Part model, mm, in its own coordinate system. Face numbers are marked on the shaded views. A direction names the side the tool comes from. Coordinates: 2 decimals unless noted, no trailing zeros. Order: outer loops, then holes, each group sorted by start corner. A loop starts at its lowest first (then second) coordinate and runs counter-clockwise, first axis right, second up.
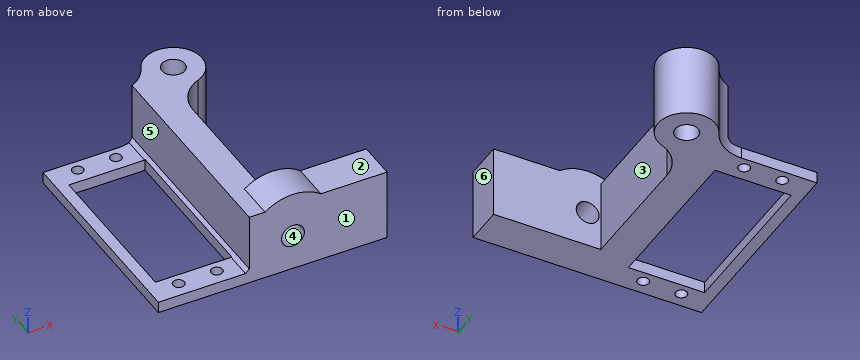
```python
from build123d import *

# Parameters (mm, degrees)
ESQUISSE1_W             = 60
ESQUISSE1_H             = 56
ESQUISSE1_W_2           = 20
ESQUISSE1_H_2           = 42
BOSS_EXTRU_1_DEPTH      = 3
ESQUISSE2_R             = 1.5
ENL_V_MAT_EXTRU_2_DEPTH = 83.127948958
BOSS_EXTRU_2_DEPTH      = 16
ESQUISSE4_W             = 28.138132954
ESQUISSE4_H             = 46
ENL_V_MAT_EXTRU_3_DEPTH = 84.618179841
ESQUISSE5_R             = 7.5
ESQUISSE5_R_2           = 3
BOSS_EXTRU_3_DEPTH      = 19
CONG_1_R                = 10
CONG_2_R                = 10
BOSS_EXTRU_4_DEPTH      = 10
ESQUISSE10_R            = 3
ENL_V_MAT_EXTRU_4_DEPTH = 10
CHANFREIN1_SIZE         = 1


with BuildPart() as part:
    # Esquisse1 → Boss.-Extru.1 (new body)
    with BuildSketch(Plane.XY):
        with Locations((30, 28)):
            Rectangle(ESQUISSE1_W, ESQUISSE1_H)
        with Locations((13, 28)):
            Rectangle(ESQUISSE1_W_2, ESQUISSE1_H_2, mode=Mode.SUBTRACT)
    extrude(amount=BOSS_EXTRU_1_DEPTH)

    # Esquisse2 → Enlèv. mat.-Extru.2 (cut, through all)
    with BuildSketch(Plane.XY.offset(3)):
        with Locations((7.5, 53)):
            Circle(ESQUISSE2_R)
        with Locations((17.5, 53)):
            Circle(ESQUISSE2_R)
        with Locations((7.5, 4)):
            Circle(ESQUISSE2_R)
        with Locations((17.5, 4)):
            Circle(ESQUISSE2_R)
    extrude(amount=-ENL_V_MAT_EXTRU_2_DEPTH, mode=Mode.SUBTRACT)

    # Esquisse3 → Boss.-Extru.2 (add)
    with BuildSketch(Plane.XY.offset(3)):
        Polygon((23.861867046, 56), (31.861867046, 56), (31.861867046, 10), (60, 10), (60, 0), (23.861867046, 0), align=None)
    extrude(amount=BOSS_EXTRU_2_DEPTH)

    # Esquisse4 → Enlèv. mat.-Extru.3 (cut, through all)
    with BuildSketch(Plane.XY.offset(3)):
        with Locations((45.930933523, 33)):
            Rectangle(ESQUISSE4_W, ESQUISSE4_H)
    extrude(amount=-ENL_V_MAT_EXTRU_3_DEPTH, mode=Mode.SUBTRACT)

    # Esquisse5 → Boss.-Extru.3 (add)
    with BuildSketch(Plane(origin=(0, 0, 0), x_dir=(-1, 0, 0), z_dir=(0, 0, -1))):
        with Locations((-35.561058301, 58.5)):
            Circle(ESQUISSE5_R)
        with Locations((-35.561058301, 58.5)):
            Circle(ESQUISSE5_R_2, mode=Mode.SUBTRACT)
    extrude(amount=-BOSS_EXTRU_3_DEPTH)

    # Congé1
    cong_1_edges = [part.edges().sort_by_distance(p)[0] for p in [
        (28.489990489, 56, 9.5),
    ]]
    fillet(cong_1_edges, radius=CONG_1_R)

    # Congé2
    cong_2_edges = [part.edges().sort_by_distance(p)[0] for p in [
        (31.861867046, 51.975738811, 9.5),
    ]]
    fillet(cong_2_edges, radius=CONG_2_R)

    # Esquisse9 → Boss.-Extru.4 (add)
    with BuildSketch(Plane.XZ):
        with BuildLine():
            Line((42.649653768, 19), (27.986775469, 19))
            ThreePointArc((27.986775469, 19), (35.318214618, 21.5), (42.649653768, 19))
        make_face()
    extrude(amount=-BOSS_EXTRU_4_DEPTH)

    # Esquisse10 → Enlèv. mat.-Extru.4 (cut)
    with BuildSketch(Plane.XZ):
        with Locations(Location((35.318214618, 9.5, 0), (0, 0, 270))):
            Circle(ESQUISSE10_R)
    extrude(amount=-ENL_V_MAT_EXTRU_4_DEPTH, mode=Mode.SUBTRACT)

    # Chanfrein1
    # the kernel refuses this chamfer: 1 mm, written as the material it adds along each edge
    with BuildSketch(Plane(origin=(23.861867046, 0, 3), x_dir=(0.027495876610585623, 0, 0.9996219169112968), z_dir=(0, 1, 0))) as chanfrein1_piece_1_section:
        Polygon((CHANFREIN1_SIZE * 0.999621916911, -CHANFREIN1_SIZE * 0.0274958766106), (-CHANFREIN1_SIZE * 0.0274958766106, -CHANFREIN1_SIZE * 0.999621916911), (0, 0), align=None)
    chanfrein1_piece_1 = extrude(amount=59.456320381, mode=Mode.PRIVATE)
    chanfrein1_piece_1 = split(chanfrein1_piece_1, bisect_by=Plane(origin=(23, 3.5, 3.33918952), z_dir=(1, 0, 0)), keep=Keep.TOP, mode=Mode.PRIVATE)
    chanfrein1_piece_1 = split(chanfrein1_piece_1, bisect_by=Plane(origin=(23.549970381, 7, 3.33918952), z_dir=(0, -1, 0)), keep=Keep.TOP, mode=Mode.PRIVATE)
    add(chanfrein1_piece_1)
    with BuildSketch(Plane(origin=(23.861867046, 0, 3), x_dir=(0.027495876610585623, 0, 0.9996219169112968), z_dir=(0, 1, 0))) as chanfrein1_piece_2_section:
        Polygon((CHANFREIN1_SIZE * 0.999621916911, -CHANFREIN1_SIZE * 0.0274958766106), (-CHANFREIN1_SIZE * 0.0274958766106, -CHANFREIN1_SIZE * 0.999621916911), (0, 0), align=None)
    chanfrein1_piece_2 = extrude(amount=59.456320381, mode=Mode.PRIVATE)
    chanfrein1_piece_2 = split(chanfrein1_piece_2, bisect_by=Plane(origin=(23, 3.5, 3.018362183), z_dir=(-1, 0, 0)), keep=Keep.TOP, mode=Mode.PRIVATE)
    chanfrein1_piece_2 = split(chanfrein1_piece_2, bisect_by=Plane(origin=(22.938869919, 7, 3.018362183), z_dir=(0, -1, 0)), keep=Keep.TOP, mode=Mode.PRIVATE)
    add(chanfrein1_piece_2)
    with BuildSketch(Plane(origin=(23.861867046, 0, 3), x_dir=(0.027495876610585623, 0, 0.9996219169112968), z_dir=(0, 1, 0))) as chanfrein1_piece_3_section:
        Polygon((CHANFREIN1_SIZE * 0.999621916911, -CHANFREIN1_SIZE * 0.0274958766106), (-CHANFREIN1_SIZE * 0.0274958766106, -CHANFREIN1_SIZE * 0.999621916911), (0, 0), align=None)
    chanfrein1_piece_3 = extrude(amount=59.456320381, mode=Mode.PRIVATE)
    chanfrein1_piece_3 = split(chanfrein1_piece_3, bisect_by=Plane(origin=(23.549970381, 49, 3.33918952), z_dir=(0, -1, 0)), keep=Keep.TOP, mode=Mode.PRIVATE)
    chanfrein1_piece_3 = split(chanfrein1_piece_3, bisect_by=Plane(origin=(23, 28, 3.33918952), z_dir=(1, 0, 0)), keep=Keep.TOP, mode=Mode.PRIVATE)
    chanfrein1_piece_3 = split(chanfrein1_piece_3, bisect_by=Plane(origin=(23.549970381, 7, 3.33918952), z_dir=(0, 1, 0)), keep=Keep.TOP, mode=Mode.PRIVATE)
    add(chanfrein1_piece_3)
    with BuildSketch(Plane(origin=(23.861867046, 0, 3), x_dir=(0.027495876610585623, 0, 0.9996219169112968), z_dir=(0, 1, 0))) as chanfrein1_piece_4_section:
        Polygon((CHANFREIN1_SIZE * 0.999621916911, -CHANFREIN1_SIZE * 0.0274958766106), (-CHANFREIN1_SIZE * 0.0274958766106, -CHANFREIN1_SIZE * 0.999621916911), (0, 0), align=None)
    chanfrein1_piece_4 = extrude(amount=59.456320381, mode=Mode.PRIVATE)
    chanfrein1_piece_4 = chanfrein1_piece_4 - Plane(origin=(19.74967, 66, 3.340715055), x_dir=(0.9035079029052511, -0.42857142857142916, 0), z_dir=(0, 0, -1)) * Cylinder(10, 123, mode=Mode.PRIVATE)
    chanfrein1_piece_4 = split(chanfrein1_piece_4, bisect_by=Plane(origin=(23.552807477, 49, 3.340715055), z_dir=(0, 1, 0)), keep=Keep.TOP, mode=Mode.PRIVATE)
    chanfrein1_piece_4 = split(chanfrein1_piece_4, bisect_by=Plane(origin=(23, 52.877415303, 3.340715055), z_dir=(1, 0, 0)), keep=Keep.TOP, mode=Mode.PRIVATE)
    add(chanfrein1_piece_4)
    with BuildSketch(Plane(origin=(23.861867046, 0, 3), x_dir=(0.027495876610585623, 0, 0.9996219169112968), z_dir=(0, 1, 0))) as chanfrein1_piece_5_section:
        Polygon((CHANFREIN1_SIZE * 0.999621916911, -CHANFREIN1_SIZE * 0.0274958766106), (-CHANFREIN1_SIZE * 0.0274958766106, -CHANFREIN1_SIZE * 0.999621916911), (0, 0), align=None)
    chanfrein1_piece_5 = extrude(amount=59.456320381, mode=Mode.PRIVATE)
    chanfrein1_piece_5 = chanfrein1_piece_5 - Plane(origin=(19.74967, 66, 3.018405741), x_dir=(0.9035079029052511, -0.42857142857142916, 0), z_dir=(0, 0, -1)) * Cylinder(10, 123, mode=Mode.PRIVATE)
    chanfrein1_piece_5 = split(chanfrein1_piece_5, bisect_by=Plane(origin=(22.938951148, 49, 3.018405741), z_dir=(0, 1, 0)), keep=Keep.TOP, mode=Mode.PRIVATE)
    chanfrein1_piece_5 = split(chanfrein1_piece_5, bisect_by=Plane(origin=(23, 52.761158893, 3.018405741), z_dir=(-1, 0, 0)), keep=Keep.TOP, mode=Mode.PRIVATE)
    add(chanfrein1_piece_5)


solid = part.part
```
(1) Drop flat-ended pins along their axis: pin 1 (7 mm diameter, centred on x = 35.56, y = 58.5, fed in from +Z); pin 2 (3.5 mm diameter, centred on x = 35.32, z = 9.5, fed in from -Y); pin 3 (2 mm diameter, centred on x = 44.5, z = 3.5, fed in from +Y). Give the stop position or say it passes through.
(2) Slice it at C-C, the plane y = 30.5. Give the cut face in (x, z).
(3) Probe line 1 (Y direction, x = 7.5, z = 2.05); line 2 (X direction, y = 35, z = 2.5); line 3 (X direction, y = 41.5, z = 10.5). List the from-to ranges inside material, lowest first.
(4) Slice it at B-B, the plane x = 7.5. Give the cut face in (y, z).
(5) Slice it at A-A, the plane z = 9.5. Give the cut face in (x, y).
(6) Tool access for the marked faces 4, 5 and 6: list every direction of +Z, -Z, +X, -X, +Y, -Y with a clear straight run to the whole face (end or side of a thin tool).
(7) Pull direction Y, two halves, no side cores. Call the marked faces 1, 2 and 3: +Y half, -Y half, draft (parallel to the pull), parting line (faces both ways), or undercut.
(8) Slice it at D-D, the plane y = 4. Give the cut face in (x, z), then the cut area to 3 significant figures.
Here are the results:
1. pin 1: stops at z = 19
1. pin 2: stops at y = 47.76
1. pin 3: stops at y = 10
2. outline: (0, 0) - (3, 0) - (3, 3) - (0, 3) - close; (23, 0) - (31.86, 0) - (31.86, 19) - (23.86, 19) - (23.86, 4) - (23, 3.14) - close
3. line 1: y = 0 to 2.5, 5.5 to 7, 49 to 51.5, 54.5 to 56
3. line 2: x = 0 to 3, 23 to 31.86
3. line 3: x = 23.86 to 31.86
4. outline: (0, 0) - (2.5, 0) - (2.5, 3) - (0, 3) - close; (5.5, 0) - (7, 0) - (7, 3) - (5.5, 3) - close; (49, 0) - (51.5, 0) - (51.5, 3) - (49, 3) - close; (54.5, 0) - (56, 0) - (56, 3) - (54.5, 3) - close
5. outline: (23.86, 0) - (32.32, 0) - (32.32, 10) - (31.86, 10) - (31.86, 42.17) arc R10 cw to (38.26, 51.5) arc R7.5 ccw (long way) to (28.78, 61.71) arc R10 cw to (23.86, 56.88) - close; (38.32, 0) - (60, 0) - (60, 10) - (38.32, 10) - close; hole circle Ø6 at (35.56, 58.5)
6. face 4: -Y
6. face 5: +Z, -X, +Y, -Y
6. face 6: +Z, -Z, +X, +Y, -Y
7. face 1: -Y half
7. face 2: draft
7. face 3: undercut
8. outline: (0, 0) - (6, 0) - (6, 3) - (0, 3) - close; (9, 0) - (16, 0) - (16, 3) - (9, 3) - close; (19, 0) - (60, 0) - (60, 19) - (42.65, 19) arc R12 ccw to (27.99, 19) - (23.86, 19) - (23.86, 4) - (22.86, 3) - (19, 3) - close; hole circle Ø6 at (35.32, 9.5)
8. area: 737 mm2
